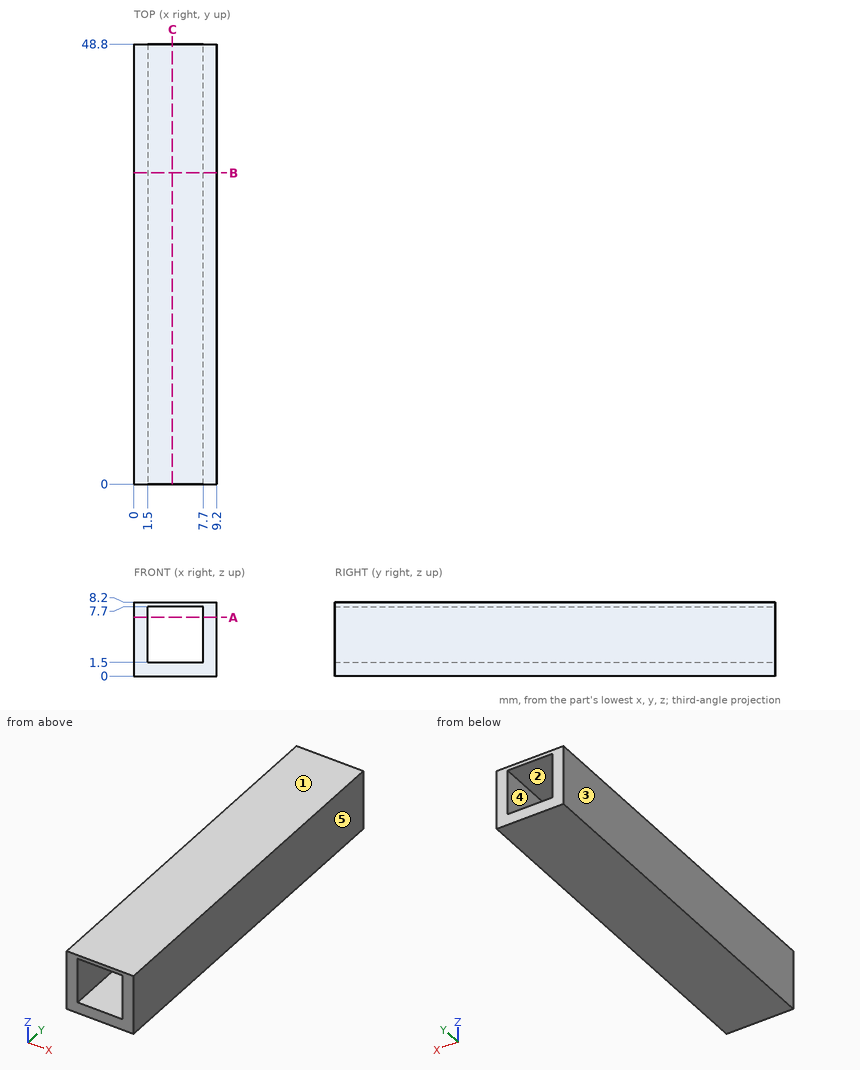
Verification items for this drawing (mm, ordinates from the low corner). A direction names the side the tool comes from. Coordinates: 2 decimals unless noted, no trailing zeros. Write each loop counter-clockwise with the first axis right and the second up, starting at its lowest first coordinate (ties: lowest second). Pieces come first, ordered by that corner, then holes. Notation, with made-up numbers: M 64.5,88 L 115.5,88 A25 ccw 115.5,117 Z; hole C 80.5,-33 d11. An arc over 180 degrees is marked long. One line per item, written item: value. Start each with the question number.
(1) Sectioned sample at C-C, the plane x = 4.25. Enter the section's corners in (y, z).
(2) Sectioned sample at B-B, the plane y = 34.5. Enter the section's corners in (x, z).
(3) Release check for a two-part mould opening along X. For the marked faces 3, 4 and 5 record: released by +X, released by -X, zero draft, split by the parting line, or undercut.
(4) Sectioned sample at A-A, the plane z = 6.5. Enter the section's corners in (x, y), and give its area (3 significant figures).
(5) Scan lines: line 1 along Z through (x, y) = (7.5, 23); line 2 along X through (y, z) = (38, 7.25). Record each from-to range of solid material in increasing order. Write a range as [from, to].
(6) Tool access check on the marked faces 1 and 2. Record the directions out of +Z, -Z, +X, -X, +Y, -Y that give a thin tool (end or side, any length) a straight path to the whole face; none if there is none.
Filled sheet:
1. outline: M 0,0 L 48.8,0 L 48.8,1.5 L 0,1.5 Z; M 0,7.7 L 48.8,7.7 L 48.8,8.2 L 0,8.2 Z
2. outline: M 0,0 L 9.2,0 L 9.2,8.2 L 0,8.2 Z; hole M 1.5,1.5 L 7.7,1.5 L 7.7,7.7 L 1.5,7.7 Z
3. face 3: released by -X
3. face 4: undercut
3. face 5: released by +X
4. outline: M 0,0 L 1.5,0 L 1.5,48.8 L 0,48.8 Z; M 7.7,0 L 9.2,0 L 9.2,48.8 L 7.7,48.8 Z
4. area: 146 mm²
5. line 1: [0, 1.5], [7.7, 8.2]
5. line 2: [0, 1.5], [7.7, 9.2]
6. face 1: +Z, +X, -X, +Y, -Y
6. face 2: +Y, -Y
